Build history of the part. All positions in model axes, mm. Face numbers are marked on the shaded views. Round coordinates to 2 decimals unless told otherwise and drop trailing zeros. Loops run counter-clockwise (first coordinate to the right, second up) from the corner with the lowest first, then second, coordinate; pieces in that order, holes last. Notation, with made-up numbers: (23, 7.5) - (47, 7.5) arc R26 ccw to (47, 38.5) - close; hole circle Ø8 at (-16, 63.5). An arc over 180 degrees is marked (long way). Use a Markdown table: item, result.
Autodesk Inventor part; units mm, degrees
ref_plane "YZ Plane" through (0, 0, 0) normal (1, 0, 0) x (0, 1, 0)
ref_plane "XZ Plane" through (0, 0, 0) normal (0, 1, 0) x (-1, 0, 0)
ref_plane "XY Plane" through (0, 0, 0) normal (0, 0, 1) x (1, 0, 0)
sketch "Sketch1" plane through (0, 0, 0) normal (0, 0, 1) x (1, 0, 0)
  line L0 (0, 0) -> (12.5, 0)
  line L1 (12.5, 0) -> (12.5, 15.5)
  line L2 (12.5, 15.5) -> (0, 15.5)
  line L3 (0, 15.5) -> (0, 0)
  dimension "d0" = 12.5
  dimension "d1" = 15.5
extrude "Extrusion1" add sketch "Sketch1" along normal blind 5.5
sketch "Sketch3" plane through (0, 0, 5.5) normal (0, 0, 1) x (1, 0, 0)
  line L0 (2.5, 2.5) -> (10, 2.5)
  line L1 (10, 2.5) -> (10, 13)
  line L2 (10, 13) -> (2.5, 13)
  line L3 (2.5, 13) -> (2.5, 2.5)
  point P0 (0, 0)
  point P1 (12, 0.5)
  point P2 (0.5, 15)
extrude "Extrusion3" cut sketch "Sketch3" against normal blind 1
sketch "Sketch5" plane through (0, 15.5, 0) normal (0, 1, 0) x (1, 0, 0)
  point P0 (0, 0)
sketch "Sketch7" plane through (0, 15.5, 0) normal (0, 1, 0) x (1, 0, 0)
  point P0 (0, 0)
sketch "Sketch8" plane through (0, 15.5, 0) normal (0, 1, 0) x (1, 0, 0)
  line L0 (0, -5.5) -> (12.5, -5.5)
  line L1 (0, 0) -> (12.5, 0)
  line L2 (12.5, 0) -> (12.5, -5.5)
  line L3 (12.5, -5.5) -> (0, -5.5)
  line L4 (0, -5.5) -> (0, 0)
  line L5 (0, 0) -> (0, -5.5)
  line L6 (12.5, 0) -> (12.5, -5.5)
  circle A0 centre (2.44, -2.75) radius 0.25
  circle A1 centre (4.98, -2.75) radius 0.25
  circle A2 centre (7.52, -2.75) radius 0.25
  circle A3 centre (10.06, -2.75) radius 0.25
  dimension "d49" = 0.5
  dimension "d50" = 0.5
  dimension "d51" = 0.5
  dimension "d52" = 0.5
extrude "Extrusion4" add sketch "Sketch8" along normal blind 8 contours A0 | A1 | A2 | A3
properties part number "DHT11"
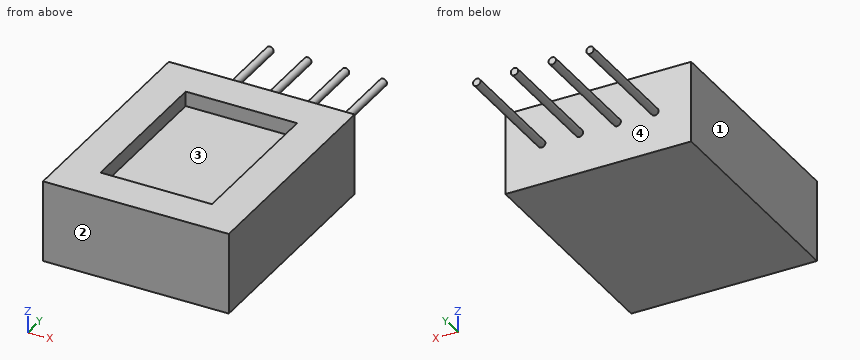
Q1. Cut at D-D, the plane y = 16.75. List the corners of the cut face in (x, z).
Results found:
| item | result |
|---|---|
| outline | circle Ø0.5 at (2.44, 2.75); circle Ø0.5 at (4.98, 2.75); circle Ø0.5 at (7.52, 2.75); circle Ø0.5 at (10.06, 2.75) |
Q2. Cut at B-B, the plane z = 2.75. List the corners of the cut face in (x, y), plus the area to 3 significant figures.
Results found:
| item | result |
|---|---|
| outline | (0, 0) - (12.5, 0) - (12.5, 15.5) - (10.31, 15.5) - (10.31, 23.5) - (9.81, 23.5) - (9.81, 15.5) - (7.77, 15.5) - (7.77, 23.5) - (7.27, 23.5) - (7.27, 15.5) - (5.23, 15.5) - (5.23, 23.5) - (4.73, 23.5) - (4.73, 15.5) - (2.69, 15.5) - (2.69, 23.5) - (2.19, 23.5) - (2.19, 15.5) - (0, 15.5) - close |
| area | 210 mm2 |
Q3. Pull direction Y, two halves, no side cores. Call the marked faces 1, 2, 3 and 4: pulls with the +Y half, pulls with the -Y half, needs draft (parallel to the pull), parting line crosses it, or undercut.
Results found:
| item | result |
|---|---|
| face 1 | needs draft |
| face 2 | pulls with the -Y half |
| face 3 | undercut |
| face 4 | pulls with the +Y half |
Q4. Drop flat-ended pins along their axis: pin 1 (4 mm diameter, centred on x = 5, y = 7, fed in from +Z); pin 2 (1.1 mm diameter, centred on x = 5, z = 5, fed in from +Y). Give the stop position or say it passes through.
Results found:
| item | result |
|---|---|
| pin 1 | stops at z = 4.5 |
| pin 2 | stops at y = 15.5 |
Q5. Probe line 1 (Y direction, x = 3, z = 4.95); line 2 (Z direction, x = 8.5, y = 11); line 3 (Y direction, x = 7.5, z = 2.4). List the from-to ranges inside material, lowest first.
Results found:
| item | result |
|---|---|
| line 1 | y = 0 to 2.5, 13 to 15.5 |
| line 2 | z = 0 to 4.5 |
| line 3 | y = 0 to 15.5 |
Q6. Cut at C-C, the plane z = 4.9. List the corners of the cut face in (x, y).
Results found:
| item | result |
|---|---|
| outline | (0, 0) - (12.5, 0) - (12.5, 15.5) - (0, 15.5) - close; hole (2.5, 2.5) - (10, 2.5) - (10, 13) - (2.5, 13) - close |
Q7. Cut at A-A, the plane x = 9.25. List the corners of the cut face in (y, z).
Results found:
| item | result |
|---|---|
| outline | (0, 0) - (15.5, 0) - (15.5, 5.5) - (13, 5.5) - (13, 4.5) - (2.5, 4.5) - (2.5, 5.5) - (0, 5.5) - close |
